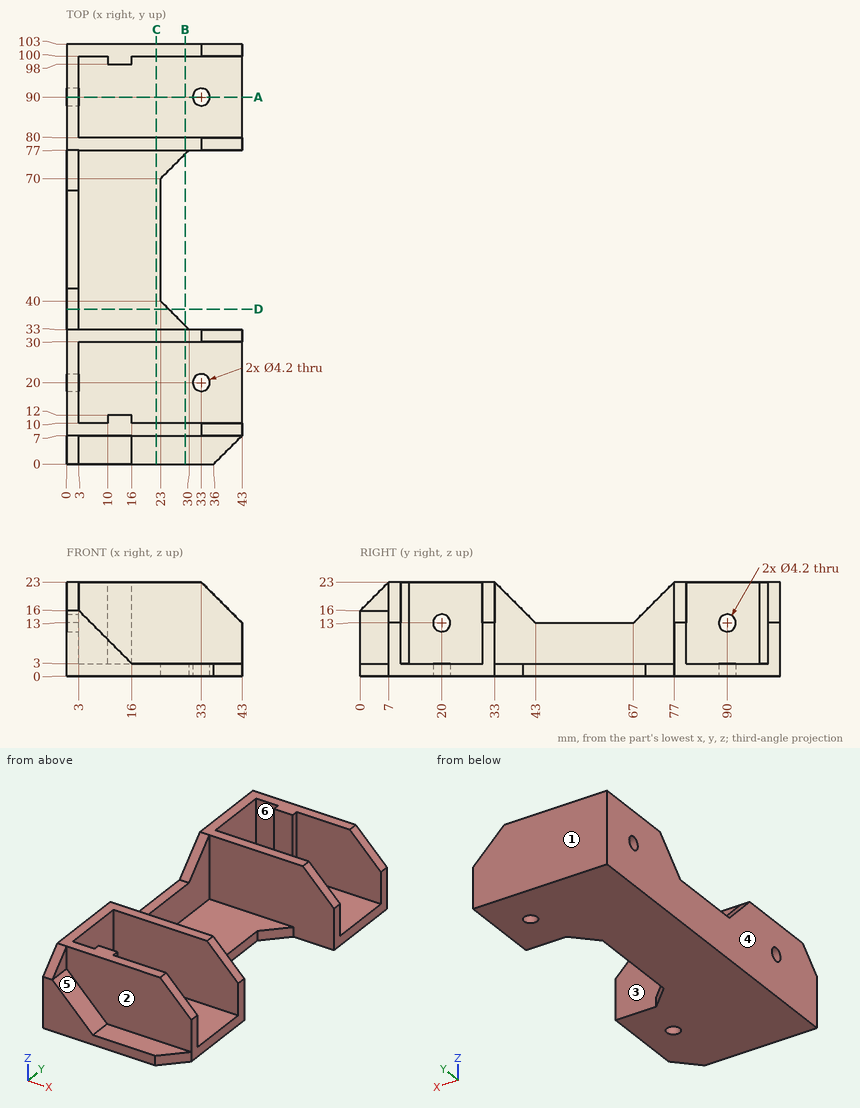
The drawing under review shows one solid part. Ordinate dimensions are in mm from its lowest x, y, z. A direction names the side the tool comes from. Coordinates: 2 decimals unless noted, no trailing zeros. Loops run counter-clockwise (first coordinate to the right, second up) from the corner with the lowest first, then second, coordinate; pieces in that order, holes last. Notation, with made-up numbers: (4, 70.5) - (23, 70.5) arc R34 ccw to (23, 103.5) - close; hole circle Ø3 at (-39.75, -17). An arc over 180 degrees is marked (long way). Use CSV: the item, a comma, the result in double quotes. Start each with the question number.
1. Add section B-B on x = 29. Give the boundary of the cut face in (y, z), plus the area to 3 significant figures.
2. Add section A-A on y = 90. Give the boundary of the cut face in (x, z).
3. For the marked faces 1, 2 and 3, list the 3-axis set-ups (+Z, -Z, +X, -X, +Y, -Y) from which the entire face can be reached by the end or side of a thin tool; tool diameter is ignored.
4. Clearance check with flat-ended pins moving along their axes: pin 1 (4 mm diameter, centred on x = 12.5, y = 54, fed in from +Z); pin 2 (5 mm diameter, centred on x = 31, z = 15.5, fed in from -Y); pin 3 (3 mm diameter, centred on y = 22.5, z = 12.5, fed in from +X). State where each tip first meets the part, or that it passes through.
5. Add section C-C on x = 22. Give the boundary of the cut face in (y, z).
6. Mouldability with a two-part tool opening along X and no side actions: class the marked faces 4, 5 and 6 as released by +X, released by -X, zero draft, split by the parting line, or undercut.
7. Add section D-D on y = 38. Give the boundary of the cut face in (x, z), plus the area to 3 significant figures.
8. To check wall thickness, follow probe 1 along Y at (x, z) = (33, 1.4); probe 2 along Y at (x, z) = (27.5, 20.75); probe 3 along Z at (x, y) = (1.15, 90). State the ranges of each line that lie inside material, in increasing order.
Resolved:
1,outline,"(0, 0) - (34, 0) - (34, 3) - (33, 3) - (33, 23) - (30, 23) - (30, 3) - (10, 3) - (10, 23) - (7, 23) - (7, 3) - (0, 3) - close; (76, 0) - (103, 0) - (103, 23) - (100, 23) - (100, 3) - (80, 3) - (80, 23) - (77, 23) - (77, 3) - (76, 3) - close"
1,area,"423 mm2"
2,outline,"(0, 0) - (30.9, 0) - (30.9, 3) - (3, 3) - (3, 10.9) - (0, 10.9) - close; (0, 15.1) - (3, 15.1) - (3, 23) - (0, 23) - close; (35.1, 0) - (43, 0) - (43, 3) - (35.1, 3) - close"
3,face 1,"+Z, -Z, +X, -X, +Y"
3,face 2,"+Z, +X, -Y"
3,face 3,"+Z, +X"
4,pin 1,"z = 3"
4,pin 2,"y = 7"
4,pin 3,"x = 3"
5,outline,"(0, 0) - (103, 0) - (103, 23) - (100, 23) - (100, 3) - (80, 3) - (80, 23) - (77, 23) - (77, 3) - (33, 3) - (33, 23) - (30, 23) - (30, 3) - (10, 3) - (10, 23) - (7, 23) - (7, 3) - (0, 3) - close"
6,face 4,"released by -X"
6,face 5,"released by +X"
6,face 6,"undercut"
7,outline,"(0, 0) - (25, 0) - (25, 3) - (3, 3) - (3, 18) - (0, 18) - close"
7,area,"120 mm2"
8,probe 1,"0 to 17.9, 22.1 to 33, 77 to 87.9, 92.1 to 103"
8,probe 2,"7 to 10, 30 to 33, 77 to 80, 100 to 103"
8,probe 3,"0 to 10.9, 15.1 to 23"
